Read the model definition and answer for the solid it produces. Units are mm, in the model's axes. Face numbers are marked on the shaded views. A direction names the side the tool comes from. Give positions to 0.01 mm unless a question says otherwise; leave off trailing zeros. Write each loop counter-clockwise with the first axis right and the second up, starting at its lowest first coordinate (ties: lowest second). Pieces come first, ordered by that corner, then holes. Notation, with made-up numbers: (27.5, 53.5) -> (82.5, 53.5) arc R7 ccw to (82.5, 61.5) -> close; hole circle Ø8 at (51.25, -19). An arc over 180 degrees is marked (long way). Answer as CSV lines item,"result". Start each with the question number.
1. The part is cut by section A-A, the plane z = -30. Determine the outline of the cut face in (x, y) (3 decimals), and give its area (3 significant figures).
2. Find the intervals of material crossed by line 1 (Z direction, x = 19.5, y = 11); line 2 (Z direction, x = 30.5, y = -4.5) (3 decimals); line 3 (Y direction, x = -38, z = -6.5), in increasing order.
3. Given pin 1 (5 mm diameter, centred on x = 8, z = -46.5, fed in from -Y); pin 2 (1.5 mm diameter, centred on x = -34, y = 13, fed in from +Z); pin 3 (2 mm diameter, centred on x = -29, z = 34.5, fed in from +Y), each flat-ended and moving along its own axis, determine where each tip first touches the part or whether it passes through.
4. For a pull along X with two mould halves and no side action, classify the marked faces 6, 7, 8 and 9 as pulls with the +X half, pulls with the -X half, needs draft (parallel to the pull), parting line crosses it, or undercut.
5. The part is cut by section B-B, the plane x = 32. Determine the outline of the cut face in (y, z) (3 decimals), and give its area (3 significant figures).
6. The part is cut by section C-C, the plane y = 29. Determine the outline of the cut face in (x, z), and give its area (3 significant figures).
7. A tool of negligible diameter and unlimited length cuts with its end or side. For the marked faces 1, 2, 3, 4 and 5, from which of +Z, -Z, +X, -X, +Y, -Y can it reach the whole face along a straight path? Write none if from no direction.
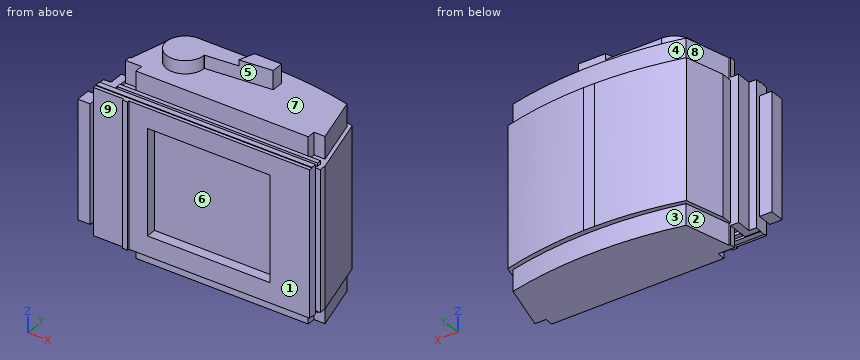
from build123d import *

# Parameters (mm, degrees)
F0_W           = 98
F0_H           = 78.35
F0_W_2         = 2.5
F0_W_3         = 16.75
F1_DEPTH       = 4.75
F2_W           = 2.75
F2_H           = 78.35
F3_DEPTH       = 1
F4_W           = 66.56
F4_H           = 56.85
F5_DEPTH       = 25
F6_W           = 117.25
F6_H           = 79
F7_DEPTH       = 2.86
F8_W           = 3.9
F8_H           = 78.35
F9_DEPTH       = 7.91
F10_W          = 8.31
F10_H          = 78.35
F11_DEPTH      = 6.5
F12_W          = 111.44
F12_H          = 75.54
F13_DEPTH      = 1.5
F14_W          = 4.41
F14_H          = 78.35
F15_DEPTH      = 9.5
F17_DEPTH      = 2.25
F19_DEPTH      = 40
F21_DEPTH      = 95.3
F23_DEPTH      = 12
F23_DEPTH_BACK = 87
F25_DEPTH      = 7
F27_DEPTH      = 3.15
F28_W          = 8
F28_H          = 63.75
F29_DEPTH      = 6.7
F30_W          = 66.56
F30_H          = 56.85
F31_DEPTH      = 5.5


with BuildPart() as f1:
    # F0 (on Front) → F1 (new body)
    with BuildSketch(Plane.XZ):
        with Locations((9.625, 0)):
            Rectangle(F0_W, F0_H)
        with Locations((-40.625, 0)):
            Rectangle(F0_W_2, F0_H)
        with Locations((-50.25, 0)):
            Rectangle(F0_W_3, F0_H)
    extrude(amount=F1_DEPTH)

    # F2 (on face) → F3 (join)
    with BuildSketch(Plane.XZ.offset(4.75)):
        with Locations((-40.75, 0)):
            Rectangle(F2_W, F2_H)
    extrude(amount=F3_DEPTH)

    # F4 (on face) → F5 (cut)
    with BuildSketch(Plane.XZ.offset(4.75)):
        with Locations((3.945, 0)):
            Rectangle(F4_W, F4_H)
    extrude(amount=-F5_DEPTH, mode=Mode.SUBTRACT)

    # F6 (on face) → F7 (join)
    with BuildSketch(Plane(origin=(0, 0, 0), x_dir=(-1, 0, 0), z_dir=(0, 1, 0))):
        Rectangle(F6_W, F6_H)
    extrude(amount=-F7_DEPTH)

    # F8 (on face) → F9 (join)
    with BuildSketch(Plane.XZ.offset(4.75)):
        with Locations((-56.675, 0)):
            Rectangle(F8_W, F8_H)
    extrude(amount=-F9_DEPTH)

    # F10 (on face) → F11 (join)
    with BuildSketch(Plane.XZ.offset(4.75)):
        with Locations((-54.47, 0)):
            Rectangle(F10_W, F10_H)
    extrude(amount=-F11_DEPTH)

    # F12 (on face) → F13 (join)
    with BuildSketch(Plane(origin=(0, 0, 0), x_dir=(-1, 0, 0), z_dir=(0, 1, 0))):
        with Locations((-5.405, -0.063661)):
            Rectangle(F12_W, F12_H)
    extrude(amount=F13_DEPTH)

    # F14 (on face) → F15 (join)
    with BuildSketch(Plane(origin=(0, 1.75, 0), x_dir=(-1, 0, 0), z_dir=(0, 1, 0))):
        with Locations((52.52, 0)):
            Rectangle(F14_W, F14_H)
    extrude(amount=F15_DEPTH)

    # F16 (on face) → F17 (join)
    with BuildSketch(Plane(origin=(0, 1.5, 0), x_dir=(-1, 0, 0), z_dir=(0, 1, 0))):
        Polygon((50.315, 39.5), (-58.625, 39.5), (-58.625, 37.706339), (-61.125, 37.706339), (-61.125, -37.833661), (-58.625, -37.833661), (-58.625, -39.5), (50.315, -39.5), align=None)
    extrude(amount=F17_DEPTH)

    # F18 (on face) → F19 (join)
    with BuildSketch(Plane(origin=(0, 3.75, 0), x_dir=(-1, 0, 0), z_dir=(0, 1, 0))):
        Polygon((-58.625, 37.706339), (-61.125, 37.706339), (-61.125, -37.833661), (-58.625, -37.833661), (50.315, -37.833661), (50.315, 37.706339), align=None)
    extrude(amount=F19_DEPTH)

    # F20 (on face) → F21 (cut)
    with BuildSketch(Plane.XY.offset(37.706339)):
        with BuildLine():
            Line((52.066333, 37.557404), (61.125, 3.75))
            Line((61.125, 3.75), (71.237857, 49.97474))
            Line((71.237857, 49.97474), (-55.704342, 49.97474))
            Line((-55.704342, 49.97474), (-51.884619, 11.25))
            Line((-51.884619, 11.25), (-44.835571, 37.557404))
            ThreePointArc((-44.835571, 37.557404), (3.615381, 43.774144), (52.066333, 37.557404))
        make_face()
    extrude(amount=-F21_DEPTH, mode=Mode.SUBTRACT)

    # F22 (on face) → F23 (join, two sides)
    with BuildSketch(Plane.XY.offset(37.706339)) as f23_sk:
        with BuildLine():
            Line((-50.315, 11.25), (-50.315, 8.25))
            Line((-50.315, 8.25), (-41.565, 8.25))
            Line((-41.565, 8.25), (-41.565, 3.75))
            Line((-41.565, 3.75), (51.919229, 3.75))
            Line((51.919229, 3.75), (51.919229, 8.25))
            Line((51.919229, 8.25), (57.919229, 8.25))
            Line((57.919229, 8.25), (50.602232, 35.557404))
            ThreePointArc((50.602232, 35.557404), (3.628124, 40.940752), (-43.345984, 35.557404))
            Line((-43.345984, 35.557404), (-49.549382, 11.25))
            Line((-49.549382, 11.25), (-50.315, 11.25))
        make_face()
    extrude(amount=F23_DEPTH)
    extrude(f23_sk.sketch, amount=-F23_DEPTH_BACK)

    # F24 (on face) → F25 (join)
    with BuildSketch(Plane.XY.offset(49.706339)):
        with BuildLine():
            ThreePointArc((-27.889039, 32.801446), (-35.316112, 15.589262), (-17.962004, 22.678382))
            ThreePointArc((-17.962004, 22.678382), (-17.963055, 22.824296), (-17.966209, 22.97018))
            ThreePointArc((-17.966209, 22.97018), (-20.960809, 29.870946), (-27.889039, 32.801446))
        make_face()
        with BuildLine():
            ThreePointArc((-27.889039, 32.801446), (-20.960809, 29.870946), (-17.966209, 22.97018))
            Line((-17.966209, 22.97018), (17.110961, 26.301446))
            Line((17.110961, 26.301446), (17.110961, 32.801446))
            Line((17.110961, 32.801446), (-27.889039, 32.801446))
        make_face()
    extrude(amount=F25_DEPTH)

    # F26 (on face) → F27 (join)
    with BuildSketch(Plane.XY.offset(56.706339)):
        Polygon((17.110961, 26.301446), (17.110961, 32.801446), (2.419159, 32.801446), (-0.427624, 24.635813), align=None)
    extrude(amount=F27_DEPTH)

    # F28 (on face) → F29 (join)
    with BuildSketch(Plane(origin=(-58.625, 0, 0), x_dir=(0, -1, 0), z_dir=(-1, 0, 0))):
        with Locations((3.34, 0)):
            Rectangle(F28_W, F28_H)
    extrude(amount=F29_DEPTH)

    # F30 (on face) → F31 (cut)
    with BuildSketch(Plane.XZ.offset(4.75)):
        with Locations((3.945, 0)):
            Rectangle(F30_W, F30_H)
    extrude(amount=-F31_DEPTH, mode=Mode.SUBTRACT)


solid = f1.part
Results found:
1,outline,"(-65.325, -7.34) -> (-58.625, -7.34) -> (-58.625, -4.75) -> (-42.125, -4.75) -> (-42.125, -5.75) -> (-39.375, -5.75) -> (-39.375, -4.75) -> (58.625, -4.75) -> (58.625, 0) -> (61.125, 0) -> (61.125, 3.75) -> (52.066, 37.557) arc R191.913 ccw to (6.659, 43.75) -> (0.571, 43.75) arc R191.913 ccw to (-44.836, 37.557) -> (-50.315, 17.108) -> (-50.315, 11.25) -> (-54.725, 11.25) -> (-54.725, 3.16) -> (-58.625, 3.16) -> (-58.625, 0.66) -> (-65.325, 0.66) -> close"
1,area,"5,050 mm²"
2,line 1,"z = -49.29 to 49.71"
2,line 2,"z = -39.175 to -28.425, 28.425 to 39.175"
2,line 3,"y = -4.75 to 39.21"
3,pin 1,"stops at y = 3.75"
3,pin 2,"stops at z = 49.71"
3,pin 3,"stops at y = 41.15"
4,face 6,"undercut"
4,face 7,"needs draft"
4,face 8,"pulls with the -X half"
4,face 9,"undercut"
5,outline,"(-4.75, -39.175) -> (-2.86, -39.175) -> (-2.86, -39.5) -> (0, -39.5) -> (0, -37.834) -> (1.5, -37.834) -> (1.5, -39.5) -> (3.75, -39.5) -> (3.75, -49.294) -> (38.993, -49.294) -> (38.993, -37.834) -> (41.663, -37.834) -> (41.663, 37.706) -> (38.993, 37.706) -> (38.993, 49.706) -> (3.75, 49.706) -> (3.75, 39.5) -> (1.5, 39.5) -> (1.5, 37.706) -> (0, 37.706) -> (0, 39.5) -> (-2.86, 39.5) -> (-2.86, 39.175) -> (-4.75, 39.175) -> (-4.75, 28.425) -> (0.75, 28.425) -> (0.75, -28.425) -> (-4.75, -28.425) -> close"
5,area,"4,040 mm²"
6,outline,"(-47.13, -37.83) -> (-45.02, -37.83) -> (-45.02, -49.29) -> (52.36, -49.29) -> (52.36, -37.83) -> (54.36, -37.83) -> (54.36, 37.71) -> (52.36, 37.71) -> (52.36, 49.71) -> (17.11, 49.71) -> (17.11, 59.86) -> (1.09, 59.86) -> (1.09, 56.71) -> (-36, 56.71) -> (-36, 49.71) -> (-45.02, 49.71) -> (-45.02, 37.71) -> (-47.13, 37.71) -> close"
6,area,"10,400 mm²"
7,face 1,"+Z, -Z, +X, -Y"
7,face 2,"-Z, -X, +Y"
7,face 3,"-Z, +Y"
7,face 4,"+Z, +Y"
7,face 5,"+Z, +X, -Y"
